Design review of the part built by this model. Coordinates are the model's own, in mm. Coordinates: 2 decimals unless noted, no trailing zeros. Write each loop counter-clockwise with the first axis right and the second up, starting at its lowest first coordinate (ties: lowest second). Pieces come first, ordered by that corner, then holes. Notation, with made-up numbers: M -29.75,87 L -13.75,87 A18 cw -13.75,101 Z; hole C -29.5,-30.75 d6. An arc over 180 degrees is marked long. Write item = value, one per line.
```python
from build123d import *

# Parameters (mm, degrees)
F0_W     = 20
F0_H     = 20
F1_DEPTH = 20
F2_R     = 9.99999
F5_D     = 5
F6_D     = 5


# Not quite as in the source:
# - a fillet or chamfer is up to 0.001 mm smaller than in the source, because OpenCascade refuses the exact size


with BuildPart() as f1:
    # F0 (on Top) → F1 (new body)
    with BuildSketch(Plane.XY):
        Rectangle(F0_W, F0_H)
    extrude(amount=F1_DEPTH)

    # F2 (radius 10 in the source; OpenCascade refuses exactly that, so slightly less here)
    f2_edges = [f1.edges().sort_by_distance(p)[0] for p in [
        (10, 0, 20),
        (-10, 0, 20),
        (0, -10, 0),
        (0, 10, 0),
    ]]
    fillet(f2_edges, radius=F2_R)

    # F5 (through all)
    with Locations(Plane(origin=(-10, 0, 0), x_dir=(0, -1, 0), z_dir=(-1, 0, 0))):
        with Locations((0, 5.5952616967)):
            Hole(F5_D / 2)

    # F6 (through all)
    with Locations(Plane.XZ.offset(10)):
        with Locations((-4.0043536574, 14.245916158), (3.62556451, 14.245916158)):
            Hole(F6_D / 2)


solid = f1.part
```
Q1. For P1, Ø3, axis at x = 1, y = 8, coming from the -Z side; P2, Ø5, axis at x = 4.5, y = 6.5, coming from the +Z side; P3, Ø8, axis at x = 8, y = -7, coming from the +Z side; P4, Ø4, axis at y = 0, z = 5.6, coming from the +X side, all flat-tipped, find the tip position at first contact; note any pin that passes through.
Check result:
P1 = 2.4
P2 = 19.8
P3 = 19.17
P4 = through
Q2. Consider section A-A, the plane x = -3.5. State how many separate pieces and enclosed holes the cut face has, and give its area (3 significant figures).
Check result:
separate_pieces = 2
enclosed_holes = 1
area = 227 mm²
Q3. Wall thickness on line 1 (X direction, y = 4.25, z = 14.25); line 2 (Z direction, x = -7.25, y = -1.75); line 3 (X direction, y = -7.5, z = 14): over which ranges is each line inside the solid? List them lowest first.
Check result:
line_1 = -9.05 to -6.5, -1.5 to 1.13, 6.13 to 9.05
line_2 = 0.15 to 3.81, 7.38 to 16.89
line_3 = -9.17 to -6.49, -1.52 to 1.14, 6.11 to 9.17
Q4. The part is to be moulded in two halves that separate along Z. For faces 1 (the flat face through (0, -10, 14)), 2 (the cylindrical face through (-3.462, 0.14, 11.805)), 3 (the cylindrical face through (7.15, 0.14, 16.99)), say which applies: +Z half, -Z half, draft (parallel to the pull), parting line (faces both ways), or undercut.
Check result:
face_1 = draft
face_2 = undercut
face_3 = +Z half
Q5. Consider section C-C, the plane z = 4.5. State the section outline as (x, y) points.
Check result:
outline = M -10,-8.35 L 10,-8.35 L 10,-2.25 L -10,-2.25 Z; M -10,2.25 L 10,2.25 L 10,8.35 L -10,8.35 Z
